from build123d import *

# Parameters (mm, degrees)
BOX001_W     = 1
BOX001_H     = 18
BOX001_DEPTH = 1
BOX_W        = 40
BOX_H        = 20
BOX_DEPTH    = 10


with BuildPart() as sphere002:
    # Sphere002 → Sphere002 (revolve)
    with BuildSketch(Plane(origin=(4, 4, 10), x_dir=(1, 0, 0), z_dir=(0, -1, 0))):
        with BuildLine():
            ThreePointArc((0, -2), (2, 0), (0, 2))
            Line((0, 2), (0, -2))
        make_face()
    revolve(axis=Axis((4, 4, 10), (0, 0, 1)))


with BuildPart() as fusion001:
    # Sphere003 → Sphere003 (revolve)
    with BuildSketch(Plane(origin=(4, 16, 10), x_dir=(1, 0, 0), z_dir=(0, -1, 0))):
        with BuildLine():
            ThreePointArc((0, -2), (2, 0), (0, 2))
            Line((0, 2), (0, -2))
        make_face()
    revolve(axis=Axis((4, 16, 10), (0, 0, 1)))

    # Fusion001: union Sphere002
    add(sphere002.part)


with BuildPart() as fusion001_1:
    # Fusion001 placement: moved
    add(fusion001.part.moved(Location((12, 0, 0))))


with BuildPart() as sphere004:
    # Sphere004 → Sphere004 (revolve)
    with BuildSketch(Plane(origin=(10, 10, 10), x_dir=(1, 0, 0), z_dir=(0, -1, 0))):
        with BuildLine():
            ThreePointArc((0, -2), (2, 0), (0, 2))
            Line((0, 2), (0, -2))
        make_face()
    revolve(axis=Axis((10, 10, 10), (0, 0, 1)))


with BuildPart() as sphere005:
    # Sphere005 → Sphere005 (revolve)
    with BuildSketch(Plane(origin=(24, 4, 10), x_dir=(1, 0, 0), z_dir=(0, -1, 0))):
        with BuildLine():
            ThreePointArc((0, -2), (2, 0), (0, 2))
            Line((0, 2), (0, -2))
        make_face()
    revolve(axis=Axis((24, 4, 10), (0, 0, 1)))


with BuildPart() as sphere007:
    # Sphere007 → Sphere007 (revolve)
    with BuildSketch(Plane(origin=(4, 16, 10), x_dir=(1, 0, 0), z_dir=(0, -1, 0))):
        with BuildLine():
            ThreePointArc((0, -2), (2, 0), (0, 2))
            Line((0, 2), (0, -2))
        make_face()
    revolve(axis=Axis((4, 16, 10), (0, 0, 1)))


with BuildPart() as sphere008:
    # Sphere008 → Sphere008 (revolve)
    with BuildSketch(Plane(origin=(36, 16, 10), x_dir=(1, 0, 0), z_dir=(0, -1, 0))):
        with BuildLine():
            ThreePointArc((0, -2), (2, 0), (0, 2))
            Line((0, 2), (0, -2))
        make_face()
    revolve(axis=Axis((36, 16, 10), (0, 0, 1)))


with BuildPart() as sphere009:
    # Sphere009 → Sphere009 (revolve)
    with BuildSketch(Plane(origin=(30, 10, 10), x_dir=(1, 0, 0), z_dir=(0, -1, 0))):
        with BuildLine():
            ThreePointArc((0, -2), (2, 0), (0, 2))
            Line((0, 2), (0, -2))
        make_face()
    revolve(axis=Axis((30, 10, 10), (0, 0, 1)))


with BuildPart() as sphere:
    # Sphere → Sphere (revolve)
    with BuildSketch(Plane(origin=(4, 4, 10), x_dir=(1, 0, 0), z_dir=(0, -1, 0))):
        with BuildLine():
            ThreePointArc((0, -2), (2, 0), (0, 2))
            Line((0, 2), (0, -2))
        make_face()
    revolve(axis=Axis((4, 4, 10), (0, 0, 1)))


with BuildPart() as fusion002:
    # Sphere001 → Sphere001 (revolve)
    with BuildSketch(Plane(origin=(4, 16, 10), x_dir=(1, 0, 0), z_dir=(0, -1, 0))):
        with BuildLine():
            ThreePointArc((0, -2), (2, 0), (0, 2))
            Line((0, 2), (0, -2))
        make_face()
    revolve(axis=Axis((4, 16, 10), (0, 0, 1)))

    # Fusion: union Sphere
    add(sphere.part)

    # Fusion002: union Fusion001, Sphere004, Sphere005, Sphere007, Sphere008, Sphere009
    add(fusion001_1.part)
    add(sphere004.part)
    add(sphere005.part)
    add(sphere007.part)
    add(sphere008.part)
    add(sphere009.part)


with BuildPart() as cube001:
    # Box001 → Box001 (new body)
    with BuildSketch(Plane(origin=(20, 1, 9), x_dir=(1, 0, 0), z_dir=(0, 0, 1))):
        with Locations((0.5, 9)):
            Rectangle(BOX001_W, BOX001_H)
    extrude(amount=BOX001_DEPTH)


with BuildPart() as cut001:
    # Box → Box (new body)
    with BuildSketch(Plane.XY):
        with Locations((20, 10)):
            Rectangle(BOX_W, BOX_H)
    extrude(amount=BOX_DEPTH)

    # Cut: cut Cube001
    add(cube001.part, mode=Mode.SUBTRACT)

    # Cut001: cut Fusion002
    add(fusion002.part, mode=Mode.SUBTRACT)


solid = cut001.part
Design review of the part built by this model. Coordinates are the model's own, in mm. A direction names the side the tool comes from. Give positions to 0.01 mm unless a question says otherwise; leave off trailing zeros. Loops run counter-clockwise (first coordinate to the right, second up) from the corner with the lowest first, then second, coordinate; pieces in that order, holes last. Notation, with made-up numbers: M 14,69 L 53,69 A12 ccw 53,90 Z; hole C 59.5,-30 d7. An arc over 180 degrees is marked long. Write item = value, one per line.
Q1. To check wall thickness, follow line 1 (X direction, y = 17, z = 9.25); line 2 (X direction, y = 5, z = 9.25); line 3 (Y direction, x = 25.5, z = 9). State the ranges of each line that lie inside material, in increasing order. Write a range as [from, to].
Output values:
line_1 = [0, 2.44], [5.56, 14.44], [17.56, 20], [21, 34.44], [37.56, 40]
line_2 = [0, 2.44], [5.56, 14.44], [17.56, 20], [21, 22.44], [25.56, 40]
line_3 = [0, 3.13], [4.87, 20]
Q2. We need section A-A (z = 9.5). Count the separate pieces of the cut face and the enclosed holes in it, plus the area to 3 significant figures.
Output values:
separate_pieces = 1
enclosed_holes = 9
area = 688 mm^2
Q3. For faces 1 (the flat face through (20, 9.9, 9.5)), 2 (the flat face through (19.7, 10.1, 10)), list the 3-axis set-ups (+Z, -Z, +X, -X, +Y, -Y) from which the entire face can be reached by the end or side of a thin tool; tool diameter is ignored.
Output values:
face_1 = +Z
face_2 = +Z, +X, -X, +Y, -Y
Q4. We need section C-C (x = 36.5). Give the boundary of the cut face in (y, z).
Output values:
outline = M 0,0 L 20,0 L 20,10 L 17.94,10 A1.94 cw 14.06,10 L 0,10 Z
Q5. We need section D-D (y = 3.5). Give the boundary of the cut face in (x, z).
Output values:
outline = M 0,0 L 40,0 L 40,10 L 25.94,10 A1.94 cw 22.06,10 L 21,10 L 21,9 L 20,9 L 20,10 L 17.94,10 A1.94 cw 14.06,10 L 5.94,10 A1.94 cw 2.06,10 L 0,10 Z
Q6. Insertion check: pin 1 (0.8 mm diameter, centred on x = 20.5, y = 14, fed in from +Z). The pin has a flat end and moves straight along its axis. Give the tip position at first contact, or say it passes through.
Output values:
pin_1 = 9
Q7. We need section B-B (y = 10.75). Give the boundary of the cut face in (x, z), plus the area to 3 significant figures.
Output values:
outline = M 0,0 L 40,0 L 40,10 L 31.85,10 A1.85 cw 28.15,10 L 21,10 L 21,9 L 20,9 L 20,10 L 11.85,10 A1.85 cw 8.15,10 L 0,10 Z
area = 388 mm^2
